Geometry check sheet. Reference: the model listing, model coordinates, mm. Face numbers are marked on the shaded views. A direction names the side the tool comes from. Round coordinates to 2 decimals unless told otherwise and drop trailing zeros. Write each loop counter-clockwise with the first axis right and the second up, starting at its lowest first coordinate (ties: lowest second). Pieces come first, ordered by that corner, then holes. Notation, with made-up numbers: (64, 11.25) - (108, 11.25) arc R24 ccw to (108, 23.25) - close; hole circle Ø4 at (-6.5, -1.75). An arc over 180 degrees is marked (long way). One line per question, with ' | ' between items. Start each with the question number.
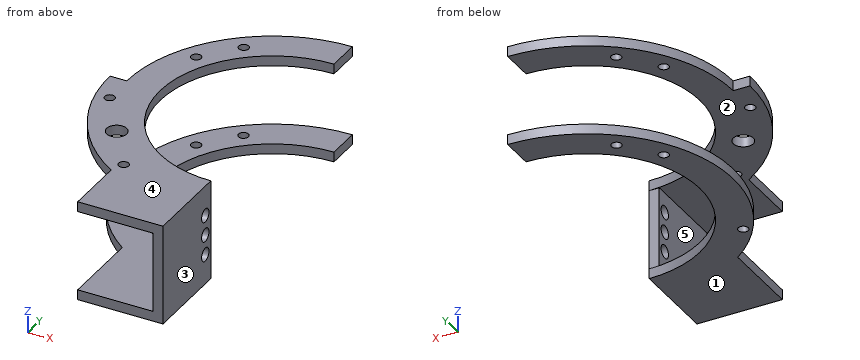
from build123d import *

# Parameters (mm, degrees)
PAD_DEPTH       = 3
SKETCH001_W     = 3
SKETCH001_H     = 26
PAD001_DEPTH    = 24
SKETCH002_R     = 2
POCKET_DEPTH    = 3
SKETCH003_R     = 1.5
SKETCH003_R_2   = 3
PAD002_DEPTH    = 3
SKETCH004_R     = 1.5
POCKET001_DEPTH = 3
SKETCH005_R     = 1.5
POCKET002_DEPTH = 30.001


with BuildPart() as part:
    # Sketch → Pad (new body)
    with BuildSketch(Plane.XY):
        with BuildLine():
            ThreePointArc((33.5, 33.5), (0, 0), (33.5, -33.5))
            Line((33.5, -33.5), (33.5, -59.5))
            Line((33.5, -59.5), (8, -59.5))
            Line((8, -59.5), (8, -35.24202))
            ThreePointArc((33.5, 43.5), (-7.884042, 13.401905), (8, -35.24202))
            Line((33.5, 33.5), (33.5, 43.5))
        make_face()
    extrude(amount=PAD_DEPTH)

    # Sketch001 → Pad001 (new body)
    with BuildSketch(Plane.XY.offset(3)):
        with Locations((32, -46.5)):
            Rectangle(SKETCH001_W, SKETCH001_H)
    extrude(amount=PAD001_DEPTH)

    # Sketch002 → Pocket (cut)
    with BuildSketch(Plane.YZ.offset(33.5)):
        with Locations((-36.5, 21)):
            Circle(SKETCH002_R)
        with Locations((-36.5, 15)):
            Circle(SKETCH002_R)
        with Locations((-36.5, 9)):
            Circle(SKETCH002_R)
    extrude(amount=-POCKET_DEPTH, mode=Mode.SUBTRACT)

    # Sketch003 → Pad002 (new body)
    with BuildSketch(Plane.XY.offset(27)):
        with BuildLine():
            Line((33.5, 43.5), (33.5, 33.5))
            ThreePointArc((33.5, 33.5), (0, 0), (33.5, -33.5))
            Line((33.5, -33.5), (33.5, -59.5))
            Line((33.5, -59.5), (8, -59.5))
            Line((8, -41.255303), (8, -59.5))
            ThreePointArc((-15, 0), (-8.861539, -23.616731), (8, -41.255303))
            Line((-15, 0), (-10, 0))
            ThreePointArc((33.5, 43.5), (2.740855, 30.759145), (-10, 0))
        make_face()
        with Locations((8.752677, 29.492711)):
            Circle(SKETCH003_R, mode=Mode.SUBTRACT)
        with Locations((-0.136024, -23.4334)):
            Circle(SKETCH003_R_2, mode=Mode.SUBTRACT)
        with Locations((-9.829466, -9.58973)):
            Circle(SKETCH003_R, mode=Mode.SUBTRACT)
        with Locations((9.557418, -37.27707)):
            Circle(SKETCH003_R, mode=Mode.SUBTRACT)
    extrude(amount=PAD002_DEPTH)

    # Sketch004 → Pocket001 (cut)
    with BuildSketch(Plane(origin=(0, 0, 0), x_dir=(1, 0, 0), z_dir=(0, 0, -1))):
        with Locations((8.68646, -29.464001)):
            Circle(SKETCH004_R)
        with Locations((-0.085234, 23.516634)):
            Circle(SKETCH004_R)
    extrude(amount=-POCKET001_DEPTH, mode=Mode.SUBTRACT)

    # Sketch005 → Pocket002 (cut, through all)
    with BuildSketch(Plane.XY.offset(30)):
        with Locations((0.158022, 19.25)):
            Circle(SKETCH005_R)
    extrude(amount=-POCKET002_DEPTH, mode=Mode.SUBTRACT)


solid = part.part
Q1. Section check D-D, the plane z = 4.5. Record the cut outline in (x, y).
Q2. Section check A-A, the plane z = 15. Record the cut outline in (x, y), then the cut area to 3 significant figures.
Q3. Go/stop test with flat-tipped pins: P1, Ø5, axis at x = 0.16, y = 19.25, coming from the -Z side; P2, Ø2.5, axis at y = -51.5, z = 28.5, coming from the -X side; P3, Ø10, axis at y = 4, z = 25, coming from the +X side; P4, Ø5, axis at y = -48, z = 12, coming from the -X side. Record where each tip stops, or that it passes through.
Q4. Draft check along Z on the marked faces 1, 2 and 3. Enter one of: pulls with the +Z half, pulls with the -Z half, needs draft (parallel to the pull), parting line crosses it, or undercut.
Q5. Thickness scan on line 1 (Z direction, x = 23, y = 35); line 2 (X direction, y = -54.5, z = 4); line 3 (Y direction, x = 10.5, z = 1). Record the ranges inside material, lowest first.
Q6. Set-up check for the marked faces 4 and 5: record each of +Z, -Z, +X, -X, +Y, -Y from which the full face is reachable in a straight line by a thin tool's end or side.
Q7. Section check C-C, the plane y = 19.25. Record the cut outline in (x, z), then the cut area to 3 significant figures.
Q8. Section check B-B, the plane y = 36.5. Record the cut outline in (x, z).
Result sheet:
1) outline: (30.5, -59.5) - (33.5, -59.5) - (33.5, -33.5) - (30.5, -33.5) - close
2) outline: (30.5, -59.5) - (33.5, -59.5) - (33.5, -38.5) - (30.5, -38.5) - close; (30.5, -34.5) - (33.5, -34.5) - (33.5, -33.5) - (30.5, -33.5) - close | area: 66.0 mm²
3) P1: z = 0 | P2: x = 8 | P3: x = 1.12 | P4: x = 30.5
4) face 1: pulls with the -Z half | face 2: undercut | face 3: needs draft
5) line 1: 0 to 3, 27 to 30 | line 2: 30.5 to 33.5 | line 3: -59.5 to -24.36, 24.36 to 36.92
6) face 4: +Z, +X, -X, +Y, -Y | face 5: -X, +Y, -Y
7) outline: (-5.51, 0) - (-1.34, 0) - (-1.34, 3) - (-5.51, 3) - close; (-5.51, 27) - (-1.34, 27) - (-1.34, 30) - (-5.51, 30) - close; (1.66, 0) - (6.08, 0) - (6.08, 3) - (1.66, 3) - close; (1.66, 27) - (6.08, 27) - (6.08, 30) - (1.66, 30) - close | area: 51.6 mm²
8) outline: (9.84, 0) - (33.5, 0) - (33.5, 3) - (9.84, 3) - close; (9.84, 27) - (33.5, 27) - (33.5, 30) - (9.84, 30) - close
